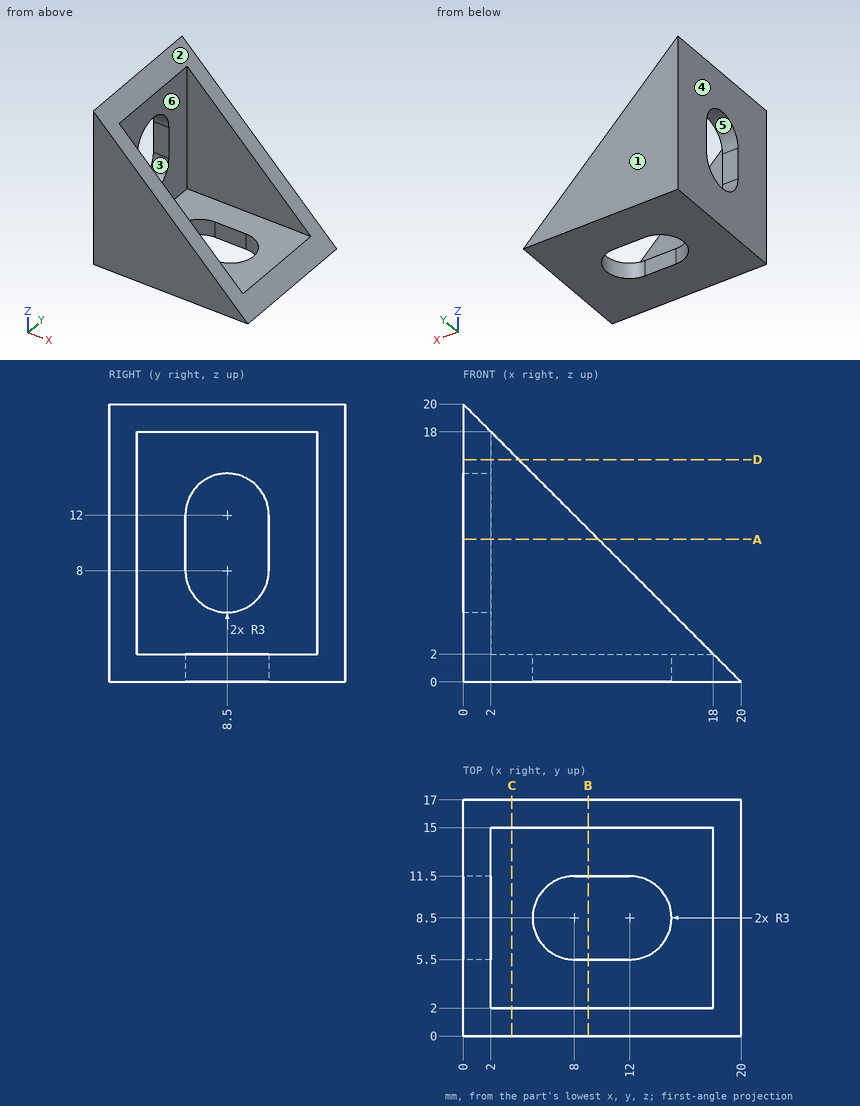
Design review of the part shown in the three views and the two pictorial views. Dimensions are in mm from the part's minimum x, y and z. A direction names the side the tool comes from. Round coordinates to 2 decimals unless told otherwise and drop trailing zeros. Write each loop counter-clockwise with the first axis right and the second up, starting at its lowest first coordinate (ties: lowest second). Pieces come first, ordered by that corner, then holes. Notation, with made-up numbers: (56.25, 40) - (80.25, 40) arc R35 cw to (80.25, 74) - close; hole circle Ø4 at (25.5, 54). An arc over 180 degrees is marked (long way). Return JSON: item names as keys, results as strings. Group by question number.
Item 1: We need section A-A on z = 10.25. Write out the cut boundary in (x, y).
Item 2: For probe 1 along Y at (x, z) = (9, 3.75); probe 2 along X at (y, z) = (11.75, 10.75), list the stretches that pass through material, from the lowest coordinate up. Write a range as [from, to].
Item 3: Machinability: for the marked faces 4, 5 and 6, which of the approach directions +Z, -Z, +X, -X, +Y, -Y give a long, thin tool a straight path to every point of the face, cutting with its end or side? Answer none if there is none.
Item 4: The part is to be moulded in two halves that separate along Y. For the marked faces 1, 2 and 3, say which applies: pulls with the +Y half, pulls with the -Y half, needs draft (parallel to the pull), parting line crosses it, or undercut.
Item 5: We need section C-C on x = 3.5. Write out the cut boundary in (y, z), and give its area (3 significant figures).
Item 6: We need section B-B on x = 9. Write out the cut boundary in (y, z), and give its area (3 significant figures).
Item 7: We need section D-D on z = 16. Write out the cut boundary in (x, y).
Model answer:
{
 "1": {"outline": "(0, 0) - (9.75, 0) - (9.75, 2) - (2, 2) - (2, 5.5) - (0, 5.5) - close; (0, 11.5) - (2, 11.5) - (2, 15) - (9.75, 15) - (9.75, 17) - (0, 17) - close"},
 "2": {"probe 1": "y = [0, 2], [15, 17]", "probe 2": "x = [0, 2]"},
 "3": {"face 4": "+Z, -Z, -X, +Y, -Y", "face 5": "+X, -X", "face 6": "+Z, +X"},
 "4": {"face 1": "pulls with the +Y half", "face 2": "needs draft", "face 3": "undercut"},
 "5": {"outline": "(0, 0) - (17, 0) - (17, 16.5) - (15, 16.5) - (15, 2) - (2, 2) - (2, 16.5) - (0, 16.5) - close", "area": "92.0 mm²"},
 "6": {"outline": "(0, 0) - (5.5, 0) - (5.5, 2) - (2, 2) - (2, 11) - (0, 11) - close; (11.5, 0) - (17, 0) - (17, 11) - (15, 11) - (15, 2) - (11.5, 2) - close", "area": "58.0 mm²"},
 "7": {"outline": "(0, 0) - (4, 0) - (4, 2) - (2, 2) - (2, 15) - (4, 15) - (4, 17) - (0, 17) - close"}
}
